CAD build for the part. Positions are in the model's coordinates, mm. A direction names the side the tool comes from. Give positions to 0.01 mm unless a question says otherwise; leave off trailing zeros. Write each loop counter-clockwise with the first axis right and the second up, starting at its lowest first coordinate (ties: lowest second). Pieces come first, ordered by that corner, then holes. Notation, with made-up numbers: M 14.5,6.25 L 28.5,6.25 A18 cw 28.5,31.25 Z; hole C -19.75,2.5 d10. An arc over 180 degrees is marked long. One line per question, with ' | ' between items. Start each with the question number.
1. Pull direction Y, two halves, no side cores. Call faces 4 (the face through (-12.3, 6.83, 8.13)), 5 (the face through (-10.9, 0, 9)), 6 (the face through (-12.3, -6.83, 8.37)): released by +Y, released by -Y, zero draft, split by the parting line, or undercut.
2. Cut at C-C, the plane x = 6. Write the cut outline in (y, z).
3. Cut at B-B, the plane z = 15.25. Write the cut outline in (x, y).
4. Wall check: L1, parallel to X at y = 0.25, z = 5.75; L2, parallel to Y at x = 1.5, z = 2.25; L3, parallel to Y at x = 2, z = 10.75. Give the ranges that are in metal, low to high.
5. Cut at D-D, the plane y = -0.75. Write the cut outline in (x, z) (3 decimals).
6. Cut at A-A, the plane z = 6.25. Write the cut outline in (x, y), then the cut area to 3 significant figures.
7. Which spindle directions (+Z, -Z, +X, -X, +Y, -Y) get a long thin tool onto all of the face, cutting with end or side? Do faces 1 (the face through (-8.65, 2.56, 8.7)), 2 (the face through (-0.075, -1, 13)), 3 (the face through (12.33, 6.8, 8.13)). Say none if no direction does.
8. Flat gauge pins, fed straight in: pin 1 (0.5 mm diameter, centred on x = 0, y = 2.5, fed in from +Z); pin 2 (2 mm diameter, centred on x = -4, y = 0, fed in from +Z). Where does each tip first touch, or does it go through?
```python
from build123d import *

# Parameters (mm, degrees)
F0_W      = 25.8
F0_H      = 14.8
F1_DEPTH  = 2
F2_W      = 25.8
F2_H      = 14.8
F2_W_2    = 21.8
F2_H_2    = 10.8
F3_DEPTH  = 14.5
F4_W      = 17.8
F4_H      = 6.8
F5_DEPTH  = 12.5
F7_DEPTH  = 17.8
F8_SIZE   = 0.5
F9_R      = 2
F10_W     = 5
F10_H     = 4
F11_DEPTH = 6
F12_W     = 17.8
F12_H     = 0.5
F12_H_2   = 2
F13_DEPTH = 1.8


with BuildPart() as f1:
    # F0 (on Top) → F1 (new body)
    with BuildSketch(Plane.XY):
        Rectangle(F0_W, F0_H)
    extrude(amount=F1_DEPTH)

    # F2 (on face) → F3 (join)
    with BuildSketch(Plane.XY.offset(2)):
        Rectangle(F2_W, F2_H)
        Rectangle(F2_W_2, F2_H_2, mode=Mode.SUBTRACT)
    extrude(amount=F3_DEPTH)

    # F4 (on face) → F5 (join)
    with BuildSketch(Plane.XY.offset(2)):
        Rectangle(F4_W, F4_H)
    extrude(amount=F5_DEPTH)

    # F6 (on face) → F7 (cut)
    with BuildSketch(Plane.YZ.offset(8.9)):
        Polygon((2.2, 2.000455), (3.4, 2), (3.4, 10), (2.2, 7.250455), align=None)
    extrude(amount=-F7_DEPTH, mode=Mode.SUBTRACT)

    # F8
    f8_edges = [f1.edges().sort_by_distance(p)[0] for p in [
        (0, 3.4, 14.5),
        (-8.9, 0, 14.5),
        (0, -3.4, 14.5),
        (8.9, 0, 14.5),
        (-8.9, -3.4, 8.25),
        (8.9, -3.4, 8.25),
        (8.9, 3.4, 12.25),
        (-8.9, 3.4, 12.25),
        (-8.9, 2.2, 4.625455),
        (-8.9, 2.8, 8.625227),
        (8.9, 2.2, 4.625455),
        (8.9, 2.8, 8.625227),
    ]]
    chamfer(f8_edges, length=F8_SIZE)

    # F9
    f9_edges = [f1.edges().sort_by_distance(p)[0] for p in [
        (-12.9, 7.4, 8.25),
        (12.9, 7.4, 8.25),
        (10.9, 5.4, 9.25),
        (-10.9, 5.4, 9.25),
        (10.9, -5.4, 9.25),
        (-10.9, -5.4, 9.25),
        (-12.9, -7.4, 8.25),
        (12.9, -7.4, 8.25),
    ]]
    fillet(f9_edges, radius=F9_R)

    # F10 (on face) → F11 (cut)
    with BuildSketch(Plane.XY.offset(16.5)):
        Polygon((-7.575, 1), (-7.575, -2), (-0.075, -2), (-0.075, 1), (-1.325, 1), (-1.325, 2), (-6.325, 2), (-6.325, 1), align=None)
        with Locations((5.075, 0)):
            Rectangle(F10_W, F10_H)
    extrude(amount=-F11_DEPTH, mode=Mode.SUBTRACT)

    # F12 (on face) → F13 (cut)
    with BuildSketch(Plane.XY.offset(2)):
        with Locations((0, -3.15)):
            Rectangle(F12_W, F12_H)
        with Locations((0, -4.4)):
            Rectangle(F12_W, F12_H_2)
    extrude(amount=-F13_DEPTH, mode=Mode.SUBTRACT)


solid = f1.part
```
Here are the results:
1) face 4: released by +Y | face 5: undercut | face 6: released by -Y
2) outline: M -7.4,0 L 7.4,0 L 7.4,16.5 L 5.4,16.5 L 5.4,2 L 3.4,2 L 2.2,2 L 2.2,7.25 L 3.4,10 L 3.4,14 L 2.9,14.5 L 2,14.5 L 2,10.5 L -2,10.5 L -2,14.5 L -2.9,14.5 L -3.4,14 L -3.4,2 L -2.9,2 L -2.9,0.2 L -5.4,0.2 L -5.4,16.5 L -7.4,16.5 Z
3) outline: M -12.9,-5.4 A2 ccw -10.9,-7.4 L 10.9,-7.4 A2 ccw 12.9,-5.4 L 12.9,5.4 A2 ccw 10.9,7.4 L -10.9,7.4 A2 ccw -12.9,5.4 Z; hole M -10.9,-3.4 A2 ccw -8.9,-5.4 L 8.9,-5.4 A2 ccw 10.9,-3.4 L 10.9,3.4 A2 ccw 8.9,5.4 L -8.9,5.4 A2 ccw -10.9,3.4 Z
4) L1: -12.9 to -10.9, -8.9 to 8.9, 10.9 to 12.9 | L2: -7.4 to -5.4, -3.4 to 2.2, 5.4 to 7.4 | L3: -7.4 to -5.4, -3.4 to 3.4, 5.4 to 7.4
5) outline: M -12.9,0 L 12.9,0 L 12.9,16.5 L 10.9,16.5 L 10.9,2 L 8.9,2 L 8.9,14 L 8.4,14.5 L 7.575,14.5 L 7.575,10.5 L 2.575,10.5 L 2.575,14.5 L -0.075,14.5 L -0.075,10.5 L -7.575,10.5 L -7.575,14.5 L -8.4,14.5 L -8.9,14 L -8.9,2 L -10.9,2 L -10.9,16.5 L -12.9,16.5 Z
6) outline: M -12.9,-5.4 A2 ccw -10.9,-7.4 L 10.9,-7.4 A2 ccw 12.9,-5.4 L 12.9,5.4 A2 ccw 10.9,7.4 L -10.9,7.4 A2 ccw -12.9,5.4 Z; M -8.9,-2.9 L -8.4,-3.4 L 8.4,-3.4 L 8.9,-2.9 L 8.9,1.7 L 8.4,2.2 L -8.4,2.2 L -8.9,1.7 Z; hole M -10.9,-3.4 A2 ccw -8.9,-5.4 L 8.9,-5.4 A2 ccw 10.9,-3.4 L 10.9,3.4 A2 ccw 8.9,5.4 L -8.9,5.4 A2 ccw -10.9,3.4 Z | area: 246 mm^2
7) face 1: none | face 2: +Z | face 3: +Z, -Z, +X, +Y
8) pin 1: z = 14.5 | pin 2: z = 10.5
